Source: three-view drawing plus pictorial views. Frame: mm from the lowest corner of the part. A direction names the side the tool comes from. Coordinates: 2 decimals unless noted, no trailing zeros. Write each loop counter-clockwise with the first axis right and the second up, starting at its lowest first coordinate (ties: lowest second). Pieces come first, ordered by that corner, then holes. Notation, with made-up numbers: (75, -26.75) - (80, -26.75) arc R27 cw to (80, -2.75) - close; hole circle Ø8 at (69.25, 30). An arc over 180 degrees is marked (long way). One line per item, written item: value.
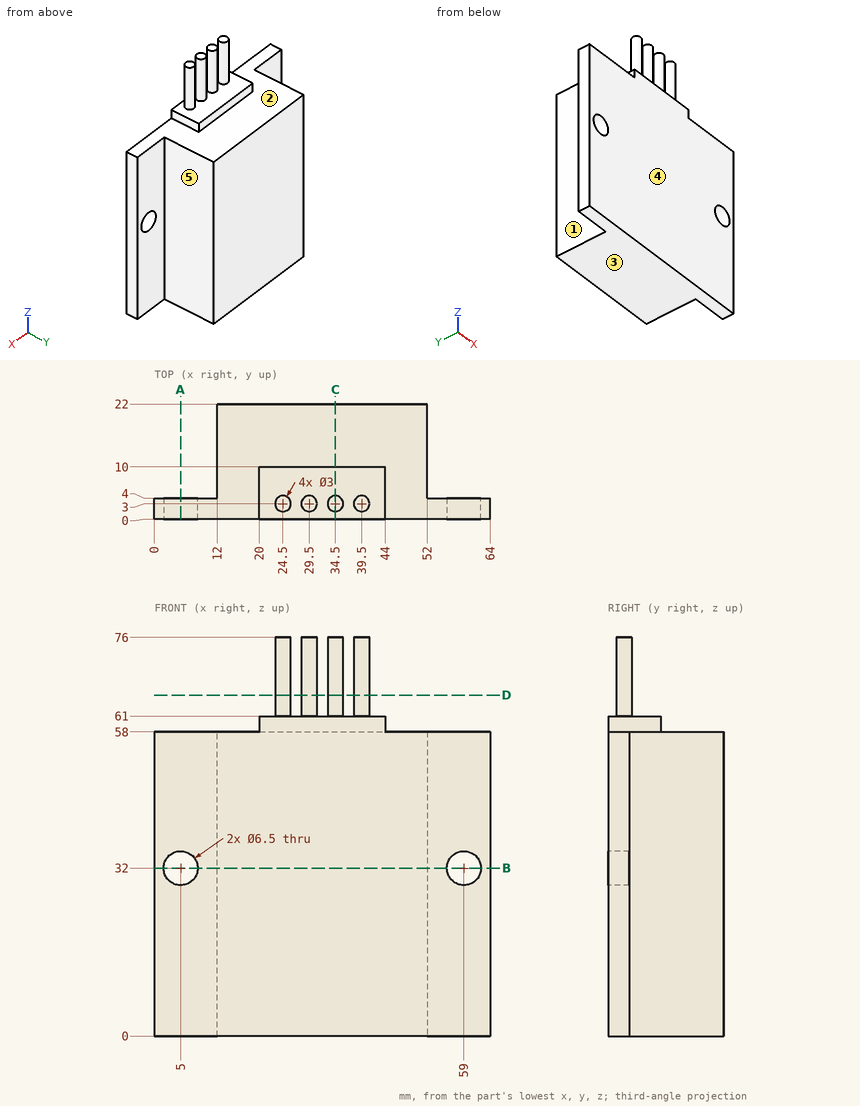
1) Section query C-C on x = 34.5. Output: boundary loops of the cut face in (y, z).
Values found:
outline: (0, 0) - (22, 0) - (22, 58) - (10, 58) - (10, 61) - (4.5, 61) - (4.5, 76) - (1.5, 76) - (1.5, 61) - (0, 61) - close
2) Contact query for flat-ended pins moving along their axis: P1, Ø3, axis at x = 28.5, y = 6.5, coming from the +Z side; P2, Ø6, axis at x = 3, z = 33.5, coming from the +Y side; P3, Ø2.5, axis at x = 32.5, z = 60, coming from the +Y side. Output: stop coordinate, or through.
Values found:
P1: z = 61
P2: y = 4
P3: y = 10
3) Reachability of the marked faces 1, 2, 3, 4 and 5 from +Z, -Z, +X, -X, +Y, -Y: full face, straight path, thin tool, end or side. Return the list, or none.
Values found:
face 1: +Z, -Z, -X, +Y
face 2: +Z, +Y
face 3: -Z, +X, -X, +Y, -Y
face 4: +Z, -Z, +X, -X, -Y
face 5: +Z, -Z, +X, +Y
4) Material intervals for line 1 (X direction, y = 2.3, z = 32); line 2 (Z direction, x = 5, y = 2.55); line 3 (X direction, y = 2.5, z = 70.5), sorted ascending.
Values found:
line 1: 0 to 1.75, 8.25 to 55.75, 62.25 to 64
line 2: 0 to 28.75, 35.25 to 58
line 3: 23.09 to 25.91, 28.09 to 30.91, 33.09 to 35.91, 38.09 to 40.91
5) Section query A-A on x = 5. Output: boundary loops of the cut face in (y, z), then the cut area to 3 significant figures.
Values found:
outline: (0, 0) - (4, 0) - (4, 28.75) - (0, 28.75) - close; (0, 35.25) - (4, 35.25) - (4, 58) - (0, 58) - close
area: 206 mm2
6) Section query D-D on z = 65. Output: boundary loops of the cut face in (x, y), then the cut area to 3 significant figures.
Values found:
outline: circle Ø3 at (24.5, 3); circle Ø3 at (29.5, 3); circle Ø3 at (34.5, 3); circle Ø3 at (39.5, 3)
area: 28.3 mm2
7) Section query B-B on z = 32. Output: boundary loops of the cut face in (x, y), then the cut area to 3 significant figures.
Values found:
outline: (0, 0) - (1.75, 0) - (1.75, 4) - (0, 4) - close; (8.25, 0) - (55.75, 0) - (55.75, 4) - (52, 4) - (52, 22) - (12, 22) - (12, 4) - (8.25, 4) - close; (62.25, 0) - (64, 0) - (64, 4) - (62.25, 4) - close
area: 924 mm2
